Check sheet for the modelled part. Datum: model origin and axes. Units: mm. A direction names the side the tool comes from. Round coordinates to 2 decimals unless told otherwise and drop trailing zeros. Write each loop counter-clockwise with the first axis right and the second up, starting at its lowest first coordinate (ties: lowest second). Pieces come first, ordered by that corner, then holes. Notation, with made-up numbers: M 34.25,52 L 49.25,52 A22 cw 49.25,66 Z; hole C 42.5,30 d5. An arc over 180 degrees is marked long. Answer in a Markdown table with one row per item.
```python
from build123d import *

# Parameters (mm, degrees)
SKETCH1_W                    = 0.15
SKETCH1_H                    = 0.5
LEGS_DEPTH                   = 6.1
LEGS_2_DEPTH                 = 6.1
FILM_START                   = 5.6
SKETCH2_W                    = 0.7
SKETCH2_H                    = 5
FILM_UP_THE_CELL_SIDE_DEPTH  = 7.39
FILM_START_2                 = 12.29
SKETCH3_W                    = 11.91
SKETCH3_H                    = 5
FILM_BETWEEN_THE_CELLS_DEPTH = 0.7


with BuildPart() as part:
    # Sketch1 → Legs (new body)
    with BuildSketch(Plane(origin=(0, 0, 0), x_dir=(1, 0, 0), z_dir=(0, 1, 0))):
        with Locations((0, 0.8)):
            Rectangle(SKETCH1_W, SKETCH1_H)
    extrude(amount=LEGS_DEPTH)



with BuildPart() as body_2:
    # Sketch1 → Legs 2 (new body)
    with BuildSketch(Plane(origin=(0, 0, 0), x_dir=(1, 0, 0), z_dir=(0, 1, 0))):
        with Locations((0, -0.8)):
            Rectangle(SKETCH1_W, SKETCH1_H)
    extrude(amount=LEGS_2_DEPTH)


with BuildPart() as part_1:
    add(part.part)

    add(body_2.part)  # Film up the cell side merges body 2
    # Sketch2 → Film up the cell side (add)
    with BuildSketch(Plane(origin=(0, 0, 0), x_dir=(1, 0, 0), z_dir=(0, 1, 0)).offset(FILM_START)):
        with Locations((0.15, 0)):
            Rectangle(SKETCH2_W, SKETCH2_H)
    extrude(amount=FILM_UP_THE_CELL_SIDE_DEPTH)

    # Sketch3 → Film between the cells (add)
    with BuildSketch(Plane(origin=(0, 0, 0), x_dir=(1, 0, 0), z_dir=(0, 1, 0)).offset(FILM_START_2)):
        with Locations((-6.155, 0)):
            Rectangle(SKETCH3_W, SKETCH3_H)
    extrude(amount=FILM_BETWEEN_THE_CELLS_DEPTH)


solid = part_1.part
```
1. Section check D-D, the plane y = 10. Record the cut outline in (x, z).
Found:
| item | result |
|---|---|
| outline | M -0.2,-2.5 L 0.5,-2.5 L 0.5,2.5 L -0.2,2.5 Z |
2. Go/stop test with flat-tipped pins: pin 1 (5 mm diameter, centred on x = -4.5, y = 6.5, fed in from +Z); pin 2 (2.5 mm diameter, centred on y = 8.5, z = -0.5, fed in from -X); pin 3 (3 mm diameter, centred on y = 11, z = 0, fed in from -X); pin 4 (0.6 mm diameter, centred on y = 3.5, z = 1, fed in from +X) (3 decimals). Record where each tip stops, or that it passes through.
Found:
| item | result |
|---|---|
| pin 1 | passes through |
| pin 2 | stops at x = -0.2 |
| pin 3 | stops at x = -12.11 |
| pin 4 | stops at x = 0.075 |
3. Scan lines: L1, parallel to Y at x = -5.5, z = -2.1; L2, parallel to X at y = 11.5, z = 1.1; L3, parallel to Z at x = 0, y = 1. Record each from-to range of solid material in increasing order.
Found:
| item | result |
|---|---|
| L1 | y = 12.29 to 12.99 |
| L2 | x = -0.2 to 0.5 |
| L3 | z = -1.05 to -0.55, 0.55 to 1.05 |
4. Section check B-B, the plane z = 2.15. Record the cut outline in (x, y).
Found:
| item | result |
|---|---|
| outline | M -12.11,12.29 L -0.2,12.29 L -0.2,5.6 L 0.5,5.6 L 0.5,12.99 L -12.11,12.99 Z |
5. Access from +Z, -Z, +X, -X, +Y, -Y to the whole of each face (thin tool, end or side, straight path). Record for faces 1 (the face through (-0.2, 9, 0)), 2 (the face through (-4, 12.6, 2.5)).
Found:
| item | result |
|---|---|
| face 1 | +Z, -Z, -X, -Y |
| face 2 | +Z, +X, -X, +Y, -Y |
6. Section check A-A, the plane y = 1. Record the cut outline in (x, z) (3 decimals).
Found:
| item | result |
|---|---|
| outline | M -0.075,-1.05 L 0.075,-1.05 L 0.075,-0.55 L -0.075,-0.55 Z; M -0.075,0.55 L 0.075,0.55 L 0.075,1.05 L -0.075,1.05 Z |
7. Section check C-C, the plane x = -7.5. Record the cut outline in (y, z).
Found:
| item | result |
|---|---|
| outline | M 12.29,-2.5 L 12.99,-2.5 L 12.99,2.5 L 12.29,2.5 Z |
